Model file for the job. Use its own axes, mm. Face numbers are marked on the shaded views. A direction names the side the tool comes from. Coordinates: 2 decimals unless noted, no trailing zeros. Write each loop counter-clockwise with the first axis right and the second up, starting at its lowest first coordinate (ties: lowest second). Pieces come first, ordered by that corner, then holes.
Q1. Pull direction Y, two halves, no side cores. Call the marked faces 1, 2 and 3: released by +Y, released by -Y, zero draft, split by the parting line, or undercut.
Q2. Band-saw the part on C-C, the plane y = -1.5. State how many separate pieces and enclosed holes the cut face has, plus the area to 3 significant figures.
Q3. Band-saw the part on B-B, the plane x = 17.5. Write the cut outline in (y, z).
Q4. Drill centre lines: probe 1 along Y at (x, z) = (-12.5, 2.15); probe 2 along Y at (x, z) = (12.5, 0.65); probe 3 along X at (y, z) = (-1.75, 5). Where is each one in solid material? Low to high.
Q5. Which spindle directions (+Z, -Z, +X, -X, +Y, -Y) get a long thin tool onto all of the face, cutting with end or side? Do the marked faces 4 and 5. Say none if no direction does.
Q6. Pin check, flat tips, straight feed: P1, Ø6, axis at x = -12.5, y = 0, coming from the +Z side; P2, Ø4, axis at x = 12.5, y = 0, coming from the -Z side. Stop position of each tip, or through.
Q7. Band-saw the part on A-A, the plane x = 12.5. Write the cut outline in (y, z).
Q8. Band-saw the part on D-D, the plane z = 6.25. Write the cut outline in (x, y), plus the area to 3 significant figures.
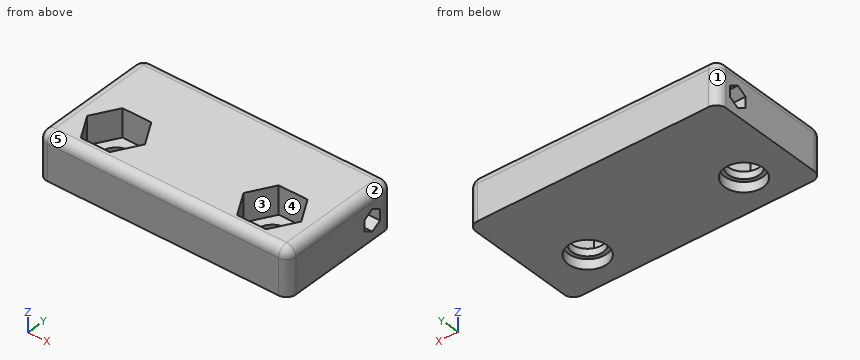
from build123d import *

# Parameters (mm, degrees)
SKETCH_W         = 40
SKETCH_H         = 20
PAD_DEPTH        = 7.25
HOLE_D           = 5
HOLE_DEPTH       = 25
HOLE_CBORE_D     = 6.2
HOLE_CBORE_DEPTH = 1.6
POCKET_DEPTH     = 4.5
POCKET001_DEPTH  = 40.001
FILLET_R         = 1.5


with BuildPart() as part:
    # Sketch → Pad (new body)
    with BuildSketch(Plane.XY):
        with Locations((0, 4)):
            Rectangle(SKETCH_W, SKETCH_H)
    extrude(amount=PAD_DEPTH)

    # Hole
    with Locations(Plane(origin=(0, 0, 0), x_dir=(1, 0, 0), z_dir=(0, 0, -1))):
        with Locations((-12.5, 0), (12.5, 0)):
            CounterBoreHole(HOLE_D / 2, HOLE_CBORE_D / 2, HOLE_CBORE_DEPTH, depth=HOLE_DEPTH)

    # Sketch002 (on Face5 of Hole) → Pocket (cut)
    with BuildSketch(Plane.XY.offset(7.25)):
        Polygon((-10.190599, 4), (-14.809401, 4), (-17.118802, 0), (-14.809401, -4), (-10.190599, -4), (-7.881198, 0), align=None)
        Polygon((10.190599, 4), (7.881198, 0), (10.190599, -4), (14.809401, -4), (17.118802, 0), (14.809401, 4), align=None)
    extrude(amount=-POCKET_DEPTH, mode=Mode.SUBTRACT)

    # Sketch003 (on Face2 of Pocket) → Pocket001 (cut, through all)
    with BuildSketch(Plane(origin=(-20, 0, 0), x_dir=(0, -1, 0), z_dir=(-1, 0, 0))):
        Polygon((-8.7, 3.866025), (-10.2, 4.732051), (-11.7, 3.866025), (-11.7, 2.133975), (-10.2, 1.267949), (-8.7, 2.133975), align=None)
    extrude(amount=-POCKET001_DEPTH, mode=Mode.SUBTRACT)

    # Fillet
    fillet_edges = [part.edges().sort_by_distance(p)[0] for p in [
        (-20, -6, 3.625),
        (-20, 4, 7.25),
        (0, 14, 7.25),
        (0, -6, 7.25),
        (-20, 14, 3.625),
        (20, 4, 7.25),
        (20, -6, 3.625),
        (20, 14, 3.625),
    ]]
    fillet(fillet_edges, radius=FILLET_R)


solid = part.part
Answer sheet:
1. face 1: released by +Y
1. face 2: zero draft
1. face 3: undercut
2. separate pieces: 3
2. enclosed holes: 0
2. area: 195 mm2
3. outline: (-6, 0) - (14, 0) - (14, 5.75) arc R1.5 ccw to (12.5, 7.25) - (-4.5, 7.25) arc R1.5 ccw to (-6, 5.75) - close; hole (8.7, 2.13) - (10.2, 1.27) - (11.7, 2.13) - (11.7, 3.87) - (10.2, 4.73) - (8.7, 3.87) - close
4. probe 1: y = -6 to -2.5, 2.5 to 8.7, 11.7 to 14
4. probe 2: y = -6 to -3.1, 3.1 to 14
4. probe 3: x = -20 to -16.11, -8.89 to 8.89, 16.11 to 20
5. face 4: +Z
5. face 5: +Z, +X, -X, -Y
6. P1: stops at z = 2.75
6. P2: passes through
7. outline: (-6, 0) - (-3.1, 0) - (-3.1, 1.6) - (-2.5, 1.6) - (-2.5, 2.75) - (-4, 2.75) - (-4, 7.25) - (-4.5, 7.25) arc R1.5 ccw to (-6, 5.75) - close; (2.5, 1.6) - (3.1, 1.6) - (3.1, 0) - (14, 0) - (14, 5.75) arc R1.5 ccw to (12.5, 7.25) - (4, 7.25) - (4, 2.75) - (2.5, 2.75) - close; hole (8.7, 2.13) - (10.2, 1.27) - (11.7, 2.13) - (11.7, 3.87) - (10.2, 4.73) - (8.7, 3.87) - close
8. outline: (-19.91, -4.5) arc R1.41 ccw to (-18.5, -5.91) - (18.5, -5.91) arc R1.41 ccw to (19.91, -4.5) - (19.91, 12.5) arc R1.41 ccw to (18.5, 13.91) - (-18.5, 13.91) arc R1.41 ccw to (-19.91, 12.5) - close; hole (-17.12, 0) - (-14.81, -4) - (-10.19, -4) - (-7.88, 0) - (-10.19, 4) - (-14.81, 4) - close; hole (7.88, 0) - (10.19, -4) - (14.81, -4) - (17.12, 0) - (14.81, 4) - (10.19, 4) - close
8. area: 677 mm2
